Geometry check sheet. Reference: the model listing, model coordinates, mm. Round coordinates to 2 decimals unless told otherwise and drop trailing zeros. Write each loop counter-clockwise with the first axis right and the second up, starting at its lowest first coordinate (ties: lowest second). Pieces come first, ordered by that corner, then holes. Notation, with made-up numbers: M -7.75,73.5 L 33.25,73.5 A29 ccw 33.25,105.5 Z; hole C 69.5,79 d9. An arc over 180 degrees is marked long. Put each result on its own line as item: value. Start each with the question number.
(1) Section check B-B on x = -21. Record the cut outline in (y, z) (3 decimals), then the cut area to 3 significant figures.
(2) Material ranges on probe 1 along Y at (x, z) = (22, 1.25) (3 decimals); probe 2 along X at (y, z) = (-13, 0.85), recorded low to high.
(3) Section check A-A on x = 0. Record the cut outline in (y, z) (3 decimals).
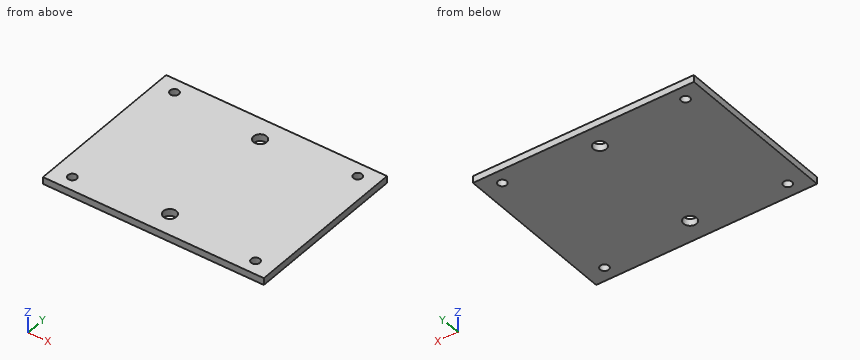
from build123d import *

# Parameters (mm, degrees)
SKETCH1_W           = 50.84
SKETCH1_H           = 38.15
SKETCH1_R           = 1.5
SKETCH1_R_2         = 1
BOSS_EXTRUDE1_DEPTH = 1.6


with BuildPart() as part:
    # Sketch1 → Boss-Extrude1 (new body)
    with BuildSketch(Plane.XY):
        Rectangle(SKETCH1_W, SKETCH1_H)
        with Locations((0, 13.975)):
            Circle(SKETCH1_R, mode=Mode.SUBTRACT)
        with Locations(Location((0, -13.975, 0), (0, 0, 180))):
            Circle(SKETCH1_R, mode=Mode.SUBTRACT)
        with Locations((-21.088938401, 15.825)):
            Circle(SKETCH1_R_2, mode=Mode.SUBTRACT)
        with Locations(Location((21.088938401, 15.825, 0), (0, 0, 180))):
            Circle(SKETCH1_R_2, mode=Mode.SUBTRACT)
        with Locations((21.088938401, -15.825)):
            Circle(SKETCH1_R_2, mode=Mode.SUBTRACT)
        with Locations(Location((-21.088938401, -15.825, 0), (0, 0, 180))):
            Circle(SKETCH1_R_2, mode=Mode.SUBTRACT)
    extrude(amount=BOSS_EXTRUDE1_DEPTH)


solid = part.part
Answers follow:
1. outline: M -19.075,0 L -16.821,0 L -16.821,1.6 L -19.075,1.6 Z; M -14.829,0 L 14.829,0 L 14.829,1.6 L -14.829,1.6 Z; M 16.821,0 L 19.075,0 L 19.075,1.6 L 16.821,1.6 Z
1. area: 54.7 mm^2
2. probe 1: y = -19.075 to -16.237, -15.413 to 15.413, 16.237 to 19.075
2. probe 2: x = -25.42 to -1.14, 1.14 to 25.42
3. outline: M -19.075,0 L -15.475,0 L -15.475,1.6 L -19.075,1.6 Z; M -12.475,0 L 12.475,0 L 12.475,1.6 L -12.475,1.6 Z; M 15.475,0 L 19.075,0 L 19.075,1.6 L 15.475,1.6 Z
